```python
from build123d import *

# Parameters (mm, degrees)
CROQUIS2_R              = 5
SALIENTE_EXTRUIR1_DEPTH = 50
CROQUIS3_W              = 10
CROQUIS3_H              = 10
SALIENTE_EXTRUIR2_DEPTH = 15
CROQUIS5_R              = 5
SALIENTE_EXTRUIR3_DEPTH = 15
CROQUIS8_R              = 0.5
SALIENTE_EXTRUIR4_DEPTH = 15
CROQUIS11_W             = 7.071067812
CROQUIS11_H             = 7.071067812
SALIENTE_EXTRUIR5_DEPTH = 7.07


with BuildPart() as part:
    # Croquis2 → Saliente-Extruir1 (new body)
    with BuildSketch(Plane.XY):
        Circle(CROQUIS2_R)
    extrude(amount=SALIENTE_EXTRUIR1_DEPTH)

    # Croquis3 → Saliente-Extruir2 (add)
    with BuildSketch(Plane.XY.offset(50)):
        Rectangle(CROQUIS3_W, CROQUIS3_H)
    extrude(amount=SALIENTE_EXTRUIR2_DEPTH)

    # Croquis5 → Saliente-Extruir3 (add)
    with BuildSketch(Plane.XZ.offset(5)):
        with Locations(Location((0, 57.5, 0), (0, 0, 180))):  # turned: the seam where the file's is
            Circle(CROQUIS5_R)
    extrude(amount=SALIENTE_EXTRUIR3_DEPTH)

    # Croquis8 → Saliente-Extruir4 (add)
    with BuildSketch(Plane.XZ.offset(20)):
        with Locations(Location((0, 57.5, 0), (0, 0, 270))):  # turned: the seam where the file's is
            Circle(CROQUIS8_R)
    extrude(amount=SALIENTE_EXTRUIR4_DEPTH)

    # Croquis11 → Saliente-Extruir5 (add)
    with BuildSketch(Plane(origin=(0, 0, 0), x_dir=(-1, 0, 0), z_dir=(0, 0, -1))):
        Rectangle(CROQUIS11_W, CROQUIS11_H)
    extrude(amount=SALIENTE_EXTRUIR5_DEPTH)


solid = part.part
```
The listing builds one solid part. Answer for the finished solid, in the listing's coordinates (mm). A direction names the side the tool comes from. Coordinates: 2 decimals unless noted, no trailing zeros. Loops run counter-clockwise (first coordinate to the right, second up) from the corner with the lowest first, then second, coordinate; pieces in that order, holes last. Notation, with made-up numbers: (-40, 45) -> (12, 45) arc R9 cw to (12, 60) -> close; hole circle Ø9 at (-10, 1.25). An arc over 180 degrees is marked (long way). Return JSON: item names as keys, results as strings. Group by question number.
(1) A cutting plane is placed at C-C on z = 28.5. Write down the section's boundary in (x, y), and give its area (3 significant figures).
(2) Given pin 1 Ø2 at (y, z) = (-3.5, 32) entering from -X; pin 2 Ø1.5 at (x, z) = (3, 30.5) entering from +Y; pin 3 Ø5.5 at (y, z) = (-0.5, -4) entering from -X; pin 4 Ø2 at (y, z) = (-6.5, 26.5) entering from +X, each flat-ended and moving along its own axis, determine where each tip first touches the part or whether it passes through.
(3) Which of the six approach directions +Z, -Z, +X, -X, +Y, -Y give full straight-line access (tool end or side, diameter ignored) to faces 1 (the flat face through (0, -5, 63)), 2 (the flat face through (0, -4, 0)), 3 (the flat face through (4, 0, 0)), 4 (the flat face through (-4, -4, 50)), 5 (the cylindrical face through (0.651, -12.395, 52.543))?
(4) A cutting plane is placed at B-B on x = 1.5. Write down the section's boundary in (y, z).
(5) Find the intervals of material crossed by probe 1 along Y at (x, z) = (-0.75, 58); probe 2 along Z at (x, y) = (-0.25, -7); probe 3 along Y at (x, z) = (3.5, 53), in increasing order. Write a range as from..to.
(6) A cutting plane is placed at A-A on y = -28. Write down the section's boundary in (x, z), and give its area (3 significant figures).
The answers:
{
 "1": {"outline": "circle Ø10 at (0, 0)", "area": "78.5 mm^2"},
 "2": {"pin 1": "stops at x = -4.33", "pin 2": "stops at y = 4.47", "pin 3": "stops at x = -3.54", "pin 4": "passes through"},
 "3": {"face 1": "+Z, -Y", "face 2": "-Z, +X, -X, -Y", "face 3": "-Z, +X, +Y, -Y", "face 4": "-Z, -X, -Y", "face 5": "-Y"},
 "4": {"outline": "(-20, 52.73) -> (-5, 52.73) -> (-5, 50) -> (-4.77, 50) -> (-4.77, 0) -> (-3.54, 0) -> (-3.54, -7.07) -> (3.54, -7.07) -> (3.54, 0) -> (4.77, 0) -> (4.77, 50) -> (5, 50) -> (5, 65) -> (-5, 65) -> (-5, 62.27) -> (-20, 62.27) -> close"},
 "5": {"probe 1": "y = -20..5", "probe 2": "z = 52.51..62.49", "probe 3": "y = -5..5"},
 "6": {"outline": "circle Ø1 at (0, 57.5)", "area": "0.785 mm^2"}
}
